For this review, take the finished solid that the model builds, in its own axes (mm). A direction names the side the tool comes from. Round coordinates to 2 decimals unless told otherwise and drop trailing zeros. Order: outer loops, then holes, each group sorted by start corner. A loop starts at its lowest first (then second) coordinate and runs counter-clockwise, first axis right, second up.
```python
from build123d import *

# Parameters (mm, degrees)
SKETCH3_R           = 1.6
BOSS_EXTRUDE1_DEPTH = 6
BOSS_EXTRUDE3_DEPTH = 40
SKETCH7_R           = 1.75
BOSS_EXTRUDE5_DEPTH = 6
CHAMFER1_SIZE       = 5
FILLET1_R           = 3
SKETCH9_R           = 19
CUT_EXTRUDE1_DEPTH  = 13.656183252


with BuildPart() as part:
    # Sketch3 → Boss-Extrude1 (new body)
    with BuildSketch(Plane.XY):
        Polygon((-42, 0), (-42, -11.15), (-57.5, -11.15), (-57.5, -3.65), (-66.6, -3.65), (-66.6, -11.15), (-82, -11.15), (-82, 0), align=None)
        with Locations((-69.5, -8.15)):
            Circle(SKETCH3_R, mode=Mode.SUBTRACT)
        with Locations((-54.5, -8.15)):
            Circle(SKETCH3_R, mode=Mode.SUBTRACT)
    extrude(amount=BOSS_EXTRUDE1_DEPTH)

    # Sketch5 → Boss-Extrude3 (add)
    with BuildSketch(Plane.ZY.offset(82)):
        Polygon((0, 0), (0, 3.464101615), (6, 0), align=None)
    extrude(amount=-BOSS_EXTRUDE3_DEPTH)

    # Sketch7 → Boss-Extrude5 (add)
    with BuildSketch(Plane(origin=(0, 4.189066469, -1.255675961), x_dir=(-1, 0, 0), z_dir=(0, 0.866025404, 0.5))):
        with Locations((78, 4.378132938)):
            Circle(SKETCH7_R)
    boss_extrude5 = extrude(amount=BOSS_EXTRUDE5_DEPTH)

    # Mirror2: Boss-Extrude5 across plane
    add(boss_extrude5.mirror(Plane(origin=(-62, 0, 0), x_dir=(0, 0, 1), z_dir=(1, 0, 0))))

    # Chamfer1
    chamfer1_edges = [part.edges().sort_by_distance(p)[0] for p in [
        (-42, -11.15, 3),
        (-82, -11.15, 3),
    ]]
    chamfer(chamfer1_edges, length=CHAMFER1_SIZE)

    # Fillet1
    fillet1_edges = [part.edges().sort_by_distance(p)[0] for p in [
        (-57.5, -11.15, 3),
        (-66.6, -11.15, 3),
    ]]
    fillet(fillet1_edges, radius=FILLET1_R)

    # Sketch9 → Cut-Extrude1 (cut, through all)
    with BuildSketch(Plane(origin=(0, 2.598076211, 1.5), x_dir=(1, 0, 0), z_dir=(0, 0.866025404, 0.5))):
        with Locations((-62, 15.803847577)):
            Circle(SKETCH9_R)
    extrude(amount=-CUT_EXTRUDE1_DEPTH, mode=Mode.SUBTRACT)


solid = part.part
```
Q1. Take a section at B-B, the plane x = -69. State the section outline as (y, z) points.
Q2. Take a section at D-D, the plane x = -51. State the section outline as (y, z) points, plus the area to 3 significant figures.
Q3. Take a section at A-A, the plane y = -9.25. State the section outline as (x, z) points, plus the area to 3 significant figures.
Q4. Tool access review of faces 4 (the face through (-62, -3.65, 3)), 5 (the face through (-77.98, 7.18, 5.56)): name each direction out of +Z, -Z, +X, -X, +Y, -Y from which nothing blocks a thin tool from reaching the whole face with its end or side.
Q5. Take a section at C-C, the plane z = 5. Count the separate pieces of the cut face and the enclosed holes in it, plus the area to 3 significant figures.
Q6. Wall thickness on line 1 (X direction, y = -6, z = 4); line 2 (Z direction, x = -45, y = -2.25); line 3 (Z direction, x = -47.5, y = 1): over which ranges is each line inside the solid? List them lowest first.
Q7. Mouldability with a two-part tool opening along Y and no side actions: class faces 1 (the face through (-67.974, -7.669, 2.958)), 2 (the face through (-73, -11.15, 3)), 3 (the face through (-66.6, -6, 3)) as +Y half, -Y half, draft (parallel to the pull), parting line (faces both ways), or undercut.
Q8. Clearance check with flat-ended pins moving along their axes: pin 1 (2.5 mm diameter, centred on x = -54.5, y = -8.15, fed in from -Z); pin 2 (9 mm diameter, centred on x = -59.5, y = -7.5, fed in from +Z); pin 3 (3.5 mm diameter, centred on y = -6.5, z = 1.5, fed in from -X); pin 4 (3 mm diameter, centred on x = -66.5, y = 0, fed in from -Z). State where each tip first meets the part, or that it passes through.
Working result:
1. outline: (-11.09, 0) - (-9.67, 0) - (-9.67, 6) - (-11.09, 6) - close; (-6.63, 0) - (-3.72, 0) - (1.67, 3.11) - (0, 6) - (-6.63, 6) - close
2. outline: (-11.15, 0) - (0.62, 0) - (2.75, 1.23) - (0, 6) - (-11.15, 6) - close
2. area: 75.5 mm2
3. outline: (-78.9, 0) - (-70.66, 0) - (-70.66, 6) - (-78.9, 6) - close; (-68.34, 0) - (-66.81, 0) - (-66.81, 6) - (-68.34, 6) - close; (-57.29, 0) - (-55.66, 0) - (-55.66, 6) - (-57.29, 6) - close; (-53.34, 0) - (-45.1, 0) - (-45.1, 6) - (-53.34, 6) - close
3. area: 118 mm2
4. face 4: +Z, -Z, -Y
4. face 5: +Z, +X, -X, +Y
5. separate pieces: 3
5. enclosed holes: 2
5. area: 384 mm2
6. line 1: x = -82 to -66.6, -57.5 to -42
6. line 2: z = 0 to 6
6. line 3: z = 0 to 4.27
7. face 1: undercut
7. face 2: -Y half
7. face 3: draft
8. pin 1: passes through
8. pin 2: stops at z = 6
8. pin 3: stops at x = -82
8. pin 4: stops at z = 2.09
